```python
from build123d import *
from build123d.topology import SkipClean

# Parameters (mm, degrees)
SKETCH1_R           = 75
SKETCH1_W           = 100
SKETCH1_H           = 100
BOSS_EXTRUDE1_DEPTH = 5
SKETCH2_R           = 8
CUT_EXTRUDE1_DEPTH  = 10
BOSS_EXTRUDE2_DEPTH = 5
BOSS_EXTRUDE4_START = -15
BOSS_EXTRUDE4_DEPTH = 15


with BuildPart() as part:
    # Sketch1 → Boss-Extrude1 (new body)
    with BuildSketch(Plane(origin=(0, 0, 0), x_dir=(1, 0, 0), z_dir=(0, 1, 0))):
        with Locations(Location((0, 0, 0), (0, 0, 270))):
            Circle(SKETCH1_R)
        Rectangle(SKETCH1_W, SKETCH1_H, mode=Mode.SUBTRACT)
    extrude(amount=BOSS_EXTRUDE1_DEPTH)

    # Sketch2 → Cut-Extrude1 (cut)
    with BuildSketch(Plane(origin=(0, 5, 0), x_dir=(1, 0, 0), z_dir=(0, 1, 0))):
        with Locations(Location((-62.5, 0, 0), (0, 0, 270))):
            Circle(SKETCH2_R)
        with Locations(Location((0, 62.5, 0), (0, 0, 270))):
            Circle(SKETCH2_R)
        with Locations(Location((62.5, 0, 0), (0, 0, 270))):
            Circle(SKETCH2_R)
        with Locations(Location((0, -62.5, 0), (0, 0, 270))):
            Circle(SKETCH2_R)
    extrude(amount=-CUT_EXTRUDE1_DEPTH, mode=Mode.SUBTRACT)

    # Sketch3 → Boss-Extrude2 (add)
    with BuildSketch(Plane(origin=(0, 5, 0), x_dir=(1, 0, 0), z_dir=(0, 1, 0))):
        with BuildLine():
            Line((50, -50), (40, -50))
            Line((40, -50), (40, -63.442887702))
            ThreePointArc((40, -63.442887702), (53.033008589, -53.033008589), (63.442887702, -40))
            Line((63.442887702, -40), (50, -40))
            Line((50, -40), (50, -50))
        make_face()
        with BuildLine():
            Line((-40, -50), (-50, -50))
            Line((-50, -50), (-50, -40))
            Line((-50, -40), (-63.442887702, -40))
            ThreePointArc((-63.442887702, -40), (-53.033008589, -53.033008589), (-40, -63.442887702))
            Line((-40, -63.442887702), (-40, -50))
        make_face()
        with BuildLine():
            Line((-63.442887702, 40), (-50, 40))
            Line((-50, 40), (-50, 50))
            Line((-50, 50), (-40, 50))
            Line((-40, 50), (-40, 63.442887702))
            ThreePointArc((-40, 63.442887702), (-53.033008589, 53.033008589), (-63.442887702, 40))
        make_face()
        with BuildLine():
            Line((50, 50), (50, 40))
            Line((50, 40), (63.442887702, 40))
            ThreePointArc((63.442887702, 40), (53.033008589, 53.033008589), (40, 63.442887702))
            Line((40, 63.442887702), (40, 50))
            Line((40, 50), (50, 50))
        make_face()
    extrude(amount=BOSS_EXTRUDE2_DEPTH)

    # Sketch4 → Boss-Extrude4 (add)
    with SkipClean():  # the faces are left unmerged after this step: merging them gives an invalid solid
        with BuildSketch(Plane(origin=(0, 10, 0), x_dir=(1, 0, 0), z_dir=(0, 1, 0)).offset(BOSS_EXTRUDE4_START)):
            with BuildLine():
                Line((50, 50), (50, 40))
                Line((50, 40), (63.442887702, 40))
                ThreePointArc((63.442887702, 40), (53.033008589, 53.033008589), (40, 63.442887702))
                Line((40, 63.442887702), (40, 50))
                Line((40, 50), (50, 50))
            make_face()
            with BuildLine():
                Line((-50, 50), (-40, 50))
                Line((-40, 50), (-40, 63.442887702))
                ThreePointArc((-40, 63.442887702), (-53.033008589, 53.033008589), (-63.442887702, 40))
                Line((-63.442887702, 40), (-50, 40))
                Line((-50, 40), (-50, 50))
            make_face()
            with BuildLine():
                Line((-40, -63.442887702), (-40, -50))
                Line((-40, -50), (-50, -50))
                Line((-50, -50), (-50, -40))
                Line((-50, -40), (-63.442887702, -40))
                ThreePointArc((-63.442887702, -40), (-53.033008589, -53.033008589), (-40, -63.442887702))
            make_face()
            with BuildLine():
                Line((50, -50), (40, -50))
                Line((40, -50), (40, -63.442887702))
                ThreePointArc((40, -63.442887702), (53.033008589, -53.033008589), (63.442887702, -40))
                Line((63.442887702, -40), (50, -40))
                Line((50, -40), (50, -50))
            make_face()
        extrude(amount=BOSS_EXTRUDE4_DEPTH)


solid = part.part
```
CAD build for the part. Positions are in the model's coordinates, mm. A direction names the side the tool comes from. Give positions to 0.01 mm unless a question says otherwise; leave off trailing zeros. Loops run counter-clockwise (first coordinate to the right, second up) from the corner with the lowest first, then second, coordinate; pieces in that order, holes last. Notation, with made-up numbers: (-37, -2) - (3, -2) arc R24 cw to (3, 22) - close; hole circle Ø8 at (79.25, -7). An arc over 180 degrees is marked (long way). Put each result on its own line as item: value.
Q1. Mould opens along Z. For faces 1 (the face through (50, -5, -51)), 2 (the face through (-4.868, 2.535, -68.849)) say: pulls with the +Z half, pulls with the -Z half, needs draft (parallel to the pull), parting line crosses it, or undercut.
Filled in:
face 1: needs draft
face 2: undercut
Q2. Slice it at A-A (z = 0). Give the cut face in (x, y).
Filled in:
outline: (-75, 0) - (-70.5, 0) - (-70.5, 5) - (-75, 5) - close; (-54.5, 0) - (-50, 0) - (-50, 5) - (-54.5, 5) - close; (50, 0) - (54.5, 0) - (54.5, 5) - (50, 5) - close; (70.5, 0) - (75, 0) - (75, 5) - (70.5, 5) - close
Q3. Slice it at D-D (z = 32). Give the cut face in (x, y).
Filled in:
outline: (-67.83, 0) - (-50, 0) - (-50, 5) - (-67.83, 5) - close; (50, 0) - (67.83, 0) - (67.83, 5) - (50, 5) - close
Q4. Tool access for faces 3 (the face through (49, -5, 52)), 4 (the face through (-40, 7, 57)), 5 (the face through (-57, 7, -40)), 6 (the face through (40, -3, -57)), 7 (the face through (1, 2, 50)): list every direction of +Z, -Z, +X, -X, +Y, -Y with a clear straight run to the whole face (end or side of a thin tool).
Filled in:
face 3: +Z, -Z, +X, -X, -Y
face 4: +Z, -Z, +Y
face 5: +X, -X, +Y
face 6: +Z, -Z, -Y
face 7: +Y, -Y
Q5. Probe line 1 along X through (y, z) = (2.85, 0); line 2 along X through (y, z) = (7.5, -51.5); line 3 along X through (y, z) = (4.75, 51.5). List the from-to ranges inside material, lowest first.
Filled in:
line 1: x = -75 to -70.5, -54.5 to -50, 50 to 54.5, 70.5 to 75
line 2: x = -54.52 to -40, 40 to 54.52
line 3: x = -54.52 to 54.52
Q6. Slice it at B-B (y = -3). Give the cut face in (x, z).
Filled in:
outline: (-63.44, -40) arc R75 ccw to (-40, -63.44) - (-40, -50) - (-50, -50) - (-50, -40) - close; (-63.44, 40) - (-50, 40) - (-50, 50) - (-40, 50) - (-40, 63.44) arc R75 ccw to start; (40, -63.44) arc R75 ccw to (63.44, -40) - (50, -40) - (50, -50) - (40, -50) - close; (40, 50) - (50, 50) - (50, 40) - (63.44, 40) arc R75 ccw to (40, 63.44) - close
Q7. Flat gauge pins, fed straight in: pin 1 (8 mm diameter, centred on x = 2, z = 57.5, fed in from -Y); pin 2 (4 mm diameter, centred on x = 52.5, y = -1.5, fed in from +Z); pin 3 (7.5 mm diameter, centred on x = -59.5, z = -8, fed in from +Y). Where does each tip first touch, or does it go through?
Filled in:
pin 1: stops at y = 0
pin 2: stops at z = 55.45
pin 3: stops at y = 5
Q8. Slice it at C-C (x = -22). Give the cut face in (y, z).
Filled in:
outline: (0, -71.7) - (5, -71.7) - (5, -50) - (0, -50) - close; (0, 50) - (5, 50) - (5, 71.7) - (0, 71.7) - close
